Autodesk Inventor part; units mm, degrees
ref_plane "YZ Plane" through (0, 0, 0) normal (1, 0, 0) x (0, 1, 0)
ref_plane "XZ Plane" through (0, 0, 0) normal (0, 1, 0) x (-1, 0, 0)
ref_plane "XY Plane" through (0, 0, 0) normal (0, 0, 1) x (1, 0, 0)
sketch "Sketch1" plane through (0, 0, 0) normal (0, 1, 0) x (-1, 0, 0)
  line L0 (82.55, 0) -> (-82.55, 0)
  line L1 (-82.55, 0) -> (-82.55, 0.0715)
  line L2 (-82.55, 0.0715) -> (-82.55, 25.4)
  line L3 (-38.1, 101.6) -> (-12.7, 101.6)
  line L4 (-12.7, 101.6) -> (-12.7, 50.8)
  line L5 (-12.7, 50.8) -> (-44.45, 50.8)
  line L6 (-44.45, 50.8) -> (-44.45, 25.4)
  line L7 (-44.45, 25.4) -> (44.45, 25.4)
  line L8 (44.45, 25.4) -> (44.45, 50.8)
  line L9 (38.1, 101.6) -> (82.55, 25.4)
  line L10 (82.55, 25.4) -> (82.55, 0)
  line L11 (38.1, 101.6) -> (12.7, 101.6)
  line L12 (12.7, 101.6) -> (12.7, 50.8)
  line L13 (12.7, 50.8) -> (44.45, 50.8)
  line L14 (0, 0) -> (0, 111.0493) construction
  line L15 (-82.55, 25.4) -> (-38.1, 101.6)
  point P0 (82.55, 12.7)
  dimension "d0" = 165.1
  dimension "d3" = 38.1
  dimension "d4" = 25.4
  dimension "d5" = 25.4
  dimension "d6" = 101.6
  dimension "d7" = 44.45
  dimension "d8" = 69.85
  dimension "d9" = 120.65
  dimension "d10" = 25.4
  dimension "d11" = 88.9
  dimension "d12" = 25.4
extrude "Extrusion1" add sketch "Sketch1" along normal blind 6.35
properties part number "Latch Clip"
Could you check a few things on this model? Use its own coordinates, in mm. A direction names the side the tool comes from. Coordinates: 2 decimals unless noted, no trailing zeros. Write each loop counter-clockwise with the first axis right and the second up, starting at its lowest first coordinate (ties: lowest second). Pieces come first, ordered by that corner, then holes. Notation, with made-up numbers: M 42.25,19.5 L 85.25,19.5 A18 cw 85.25,43.5 Z; hole C 40.5,0.5 d3. An arc over 180 degrees is marked long. Answer as CSV lines item,"result". Start each with the question number.
1) I want a section at D-D, the plane x = -2. Please give me the cut outline in (y, z), and give its area (3 significant figures).
2) We'd pull the mould along X, two halves only. Please class faces 4 (the flat face through (-60.014, 3.131, 64.033)), 5 (the flat face through (-12.7, 3, 77)), 6 (the flat face through (26, 3, 101.6)), 7 (the flat face through (1, 3, 25.4)): +X half, -X half, draft (parallel to the pull), parting line (faces both ways), or undercut.
3) I want a section at A-A, the plane z = 29. Please give me the cut outline in (x, y), and give its area (3 significant figures).
4) For P1, Ø1.5, axis at y = 3.5, z = 67.5, coming from the +X side; P2, Ø2, axis at x = -0.5, y = 1, coming from the -Z side; P3, Ø1.9, axis at y = 4, z = 65, coming from the -X side; P4, Ø3, axis at y = 4, z = 37.5, coming from the +X side, each with a flat end and sliding along its axis, tell me the tip position at first contact or that it passes through.
5) I want a section at B-B, the plane x = -30. Please give me the cut outline in (y, z).
6) Please list where these lines run through material, in increasing order: line 1 (Z direction, x = -25, y = 3.25); line 2 (Z direction, x = 2, y = 4); line 3 (X direction, y = 5, z = 68.5). Write a range as from..to.
7) For faces 1 (the flat face through (12.7, 3, 77)), 2 (the flat face through (82.55, 3, 13)), 3 (the flat face through (-28, 3, 50.8)), which set-ups out of +Z, -Z, +X, -X, +Y, -Y let a thin tool reach every point of the face, with its end or its side?
8) I want a section at C-C, the plane y = 1.5. Please give me the cut outline in (x, z).
Data:
1,outline,"M 0,0 L 6.35,0 L 6.35,25.4 L 0,25.4 Z"
1,area,"161 mm^2"
2,face 4,"-X half"
2,face 5,"undercut"
2,face 6,"draft"
2,face 7,"undercut"
3,outline,"M -80.45,0 L -44.45,0 L -44.45,6.35 L -80.45,6.35 Z; M 44.45,0 L 80.45,0 L 80.45,6.35 L 44.45,6.35 Z"
3,area,"457 mm^2"
4,P1,"stops at x = 58.43"
4,P2,"stops at z = 0"
4,P3,"stops at x = -60"
4,P4,"stops at x = 76.37"
5,outline,"M 0,0 L 6.35,0 L 6.35,25.4 L 0,25.4 Z; M 0,50.8 L 6.35,50.8 L 6.35,101.6 L 0,101.6 Z"
6,line 1,"z = 0..25.4, 50.8..101.6"
6,line 2,"z = 0..25.4"
6,line 3,"x = -57.41..-12.7, 12.7..57.41"
7,face 1,"+Z, +Y, -Y"
7,face 2,"+Z, -Z, +X, +Y, -Y"
7,face 3,"+Y, -Y"
8,outline,"M -82.55,0 L 82.55,0 L 82.55,25.4 L 38.1,101.6 L 12.7,101.6 L 12.7,50.8 L 44.45,50.8 L 44.45,25.4 L -44.45,25.4 L -44.45,50.8 L -12.7,50.8 L -12.7,101.6 L -38.1,101.6 L -82.55,25.4 Z"
